Check sheet for the modelled part. Datum: model origin and axes. Units: mm. Face numbers are marked on the shaded views. A direction names the side the tool comes from. Coordinates: 2 decimals unless noted, no trailing zeros. Loops run counter-clockwise (first coordinate to the right, second up) from the corner with the lowest first, then second, coordinate; pieces in that order, holes last.
```python
from build123d import *

# Parameters (mm, degrees)
F1_DEPTH = 5
F2_DEPTH = 15
F3_R     = 1


with BuildPart() as f1:
    # F0 (on Top) → F1 (new body)
    with BuildSketch(Plane.XY):
        with BuildLine():
            ThreePointArc((-13.7873085422, -2.4310744873), (0, -14), (13.7873085422, -2.4310744873))
            ThreePointArc((13.7873085422, -2.4310744873), (13.9467257733, -1.2201803985), (14, 0))
            ThreePointArc((14, 0), (-1.2201803985, 13.9467257733), (-13.7873085422, -2.4310744873))
        make_face()
        with BuildLine():
            Line((13.7873085422, -2.4310744873), (15.7519134057, 8.7107533578))
            ThreePointArc((15.7519134057, 8.7107533578), (0, 18), (-15.7519134057, 8.7107533578))
            Line((-15.7519134057, 8.7107533578), (-13.7873085422, -2.4310744873))
            ThreePointArc((-13.7873085422, -2.4310744873), (-1.2201803985, 13.9467257733), (14, 0))
            ThreePointArc((14, 0), (13.9467257733, -1.2201803985), (13.7873085422, -2.4310744873))
        make_face()
    extrude(amount=F1_DEPTH)

    # F0 (on Top) → F2 (join)
    with BuildSketch(Plane.XY):
        with BuildLine():
            ThreePointArc((-15.7519134057, 8.7107533578), (-4.4980861874, -17.4289190902), (18, 0))
            ThreePointArc((18, 0), (17.4289190902, 4.4980861874), (15.7519134057, 8.7107533578))
            Line((15.7519134057, 8.7107533578), (13.7873085422, -2.4310744873))
            ThreePointArc((13.7873085422, -2.4310744873), (0, -14), (-13.7873085422, -2.4310744873))
            Line((-13.7873085422, -2.4310744873), (-15.7519134057, 8.7107533578))
        make_face()
    extrude(amount=F2_DEPTH)

    # F3
    f3_edges = [f1.edges().sort_by_distance(p)[0] for p in [
        (-15.751913, 8.710753, 10),
        (15.751913, 8.710753, 10),
    ]]
    fillet(f3_edges, radius=F3_R)


solid = f1.part
```
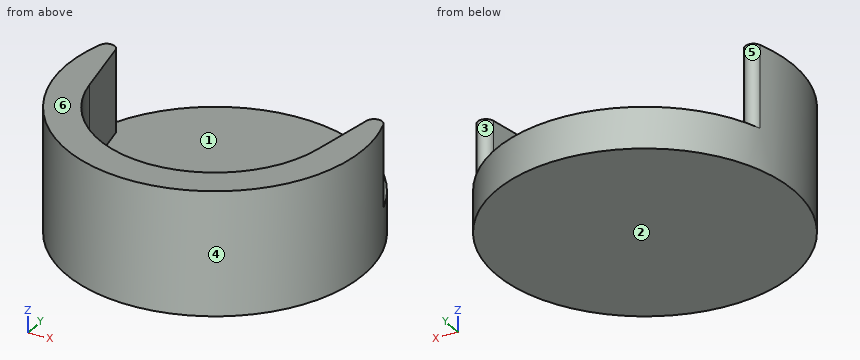
1) Set-up check for the marked faces 5 and 6: record each of +Z, -Z, +X, -X, +Y, -Y from which the full face is reachable in a straight line by a thin tool's end or side.
Answer sheet:
face 5: +Z, +Y
face 6: +Z, +X, -X, +Y, -Y
2) Section check B-B on y = 0. Enter the section's corners in (x, z).
Answer sheet:
outline: (-18, 0) - (18, 0) - (18, 15) - (14.22, 15) - (14.22, 5) - (-14.22, 5) - (-14.22, 15) - (-18, 15) - close
3) Depth check by flat-ended pin: pin 1 (6 mm diameter, centred on x = 0.5, y = -5, fed in from +Z); pin 2 (5 mm diameter, centred on y = 14.5, z = 2, fed in from +X); pin 3 (1.5 mm diameter, centred on x = 10.5, z = 4, fed in from +Y). Enter the tip coordinate at first touch or a pass-through.
Answer sheet:
pin 1: stops at z = 5
pin 2: stops at x = 13.42
pin 3: stops at y = 15.13
4) Section check A-A on x = 0. Enter the section's corners in (y, z), plus the area to 3 significant figures.
Answer sheet:
outline: (-18, 0) - (18, 0) - (18, 5) - (-14, 5) - (-14, 15) - (-18, 15) - close
area: 220 mm2
5) Mould release check, pull along X, two halves, no side actions. Record for the marked faces 1, 2, 3 and 4: +X half, -X half, draft (parallel to the pull), parting line (faces both ways), or undercut.
Answer sheet:
face 1: undercut
face 2: draft
face 3: undercut
face 4: parting line
6) Section check C-C on z = 11. Enter the section's corners in (x, y), plus the area to 3 significant figures.
Answer sheet:
outline: (-17.11, 5.58) arc R18 ccw (long way) to (17.11, 5.58) arc R1 ccw to (15.18, 5.45) - (13.79, -2.43) arc R14 cw to (-13.79, -2.43) - (-15.18, 5.45) arc R1 ccw to start
area: 236 mm2
7) Scan lines: line 1 (Z direction, x = -9, y = 14); line 2 (X direction, y = 4.5, z = 8.75); line 3 (X direction, y = -10, z = 12). Record each from-to range of solid material in increasing order.
Answer sheet:
line 1: z = 0 to 5
line 2: x = -17.43 to -15.01, 15.01 to 17.43
line 3: x = -14.97 to -9.8, 9.8 to 14.97
8) Section check D-D on z = 4. Enter the section's corners in (x, y), plus the area to 3 significant figures.
Answer sheet:
outline: circle Ø36 at (0, 0)
area: 1,020 mm2
